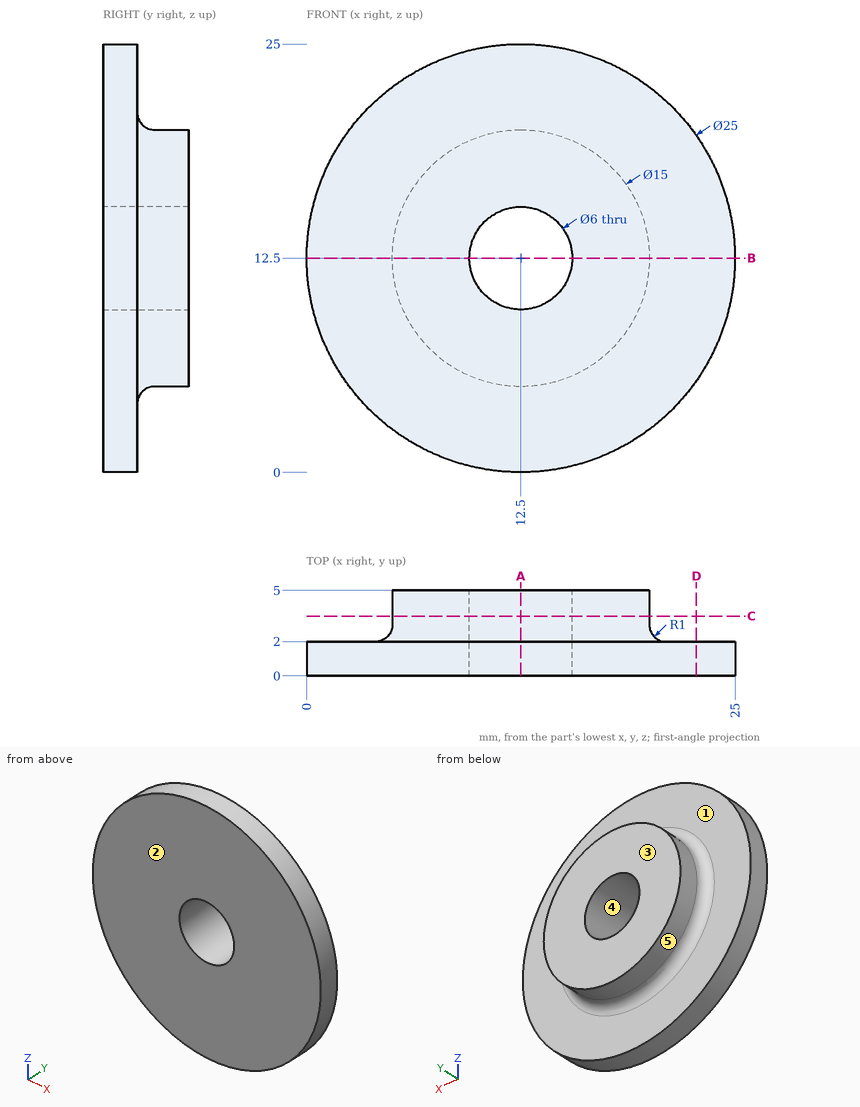
Can you work these out from the drawing? Everything is in mm from the part's minimum corner. A direction names the side the tool comes from. Give positions to 0.01 mm unless a question says otherwise; leave off trailing zeros. Loops run counter-clockwise (first coordinate to the right, second up) from the corner with the lowest first, then second, coordinate; pieces in that order, holes last. Notation, with made-up numbers: M 60,26 L 70,26 A15 ccw 70,43 Z; hole C 36.25,58.25 d5. An arc over 180 degrees is marked long. Use CSV: the item, a comma, the result in double quotes. Start each with the question number.
1. If we mould it in two halves opening along X, with no side actions, what happens to the marked faces 3, 4 and 5? For each: released by +X, released by -X, zero draft, split by the parting line, or undercut.
2. If I drill on L1, parallel to Y at x = 4, z = 4.25; L2, parallel to X at y = 1.9, z = 12.5; L3, parallel to X at y = 4.3, z = 10, over which ranges is the centre line in solid material (lowest first)?
3. Imagine slicing it at D-D, the plane x = 22.75. Write out the boundary of the cut face in (y, z), plus the area to 3 significant figures.
4. On a 3-axis mill with a long thin cutter (end or side, diameter ignored), from which of +Z, -Z, +X, -X, +Y, -Y can I reach the whole of each face in a straight line? I mean the marked faces 1 and 2. Say none if no direction works.
5. Imagine slicing it at A-A, the plane x = 12.5. Write out the boundary of the cut face in (y, z).
6. Imagine slicing it at C-C, the plane y = 3.5. Write out the boundary of the cut face in (x, z).
7. Imagine slicing it at B-B, the plane z = 12.5. Write out the boundary of the cut face in (x, y).
8. For P1, Ø1.5, axis at x = 21.5, y = 0.5, coming from the +Z side, with a flat end and sliding along its axis, tell me the tip position at first contact or that it passes through.
Response values:
1,face 3,"zero draft"
1,face 4,"undercut"
1,face 5,"split by the parting line"
2,L1,"0 to 2"
2,L2,"0 to 9.5, 15.5 to 25"
2,L3,"5.43 to 10.84, 14.16 to 19.57"
3,outline,"M 0,5.35 L 2,5.35 L 2,19.65 L 0,19.65 Z"
3,area,"28.6 mm^2"
4,face 1,"+Y"
4,face 2,"+Z, -Z, +X, -X, -Y"
5,outline,"M 0,0 L 2,0 L 2,4 A1 cw 3,5 L 5,5 L 5,9.5 L 0,9.5 Z; M 0,15.5 L 5,15.5 L 5,20 L 3,20 A1 cw 2,21 L 2,25 L 0,25 Z"
6,outline,"C 12.5,12.5 d15; hole C 12.5,12.5 d6"
7,outline,"M 0,0 L 9.5,0 L 9.5,5 L 5,5 L 5,3 A1 cw 4,2 L 0,2 Z; M 15.5,0 L 25,0 L 25,2 L 21,2 A1 cw 20,3 L 20,5 L 15.5,5 Z"
8,P1,"z = 21.89"
